```python
from build123d import *

# Parameters (mm, degrees)
SKETCH1_W           = 20
SKETCH1_H           = 20
BOSS_EXTRUDE1_DEPTH = 100
CUT_EXTRUDE1_DEPTH  = 101.995049384
CIRPATTERN1_COUNT   = 4
FILLET1_R           = 2


with BuildPart() as part:
    # Sketch1 → Boss-Extrude1 (new body)
    with BuildSketch(Plane.XY):
        Rectangle(SKETCH1_W, SKETCH1_H)
    extrude(amount=BOSS_EXTRUDE1_DEPTH)

    # Sketch2 → Cut-Extrude1 (cut, through all)
    with BuildSketch(Plane.XY):
        Polygon((6.021836642, 10), (-6.021836642, 10), (-2.5, 3.9), (2.5, 3.9), align=None)
    cut_extrude1 = extrude(amount=CUT_EXTRUDE1_DEPTH, mode=Mode.SUBTRACT)

    # CirPattern1: Cut-Extrude1 ×4 about axis
    cirpattern1_axis = Axis((0, 0, 0), (0, 0, 1))
    for i in range(1, CIRPATTERN1_COUNT):
        add(cut_extrude1.rotate(cirpattern1_axis, i * 360 / CIRPATTERN1_COUNT), mode=Mode.SUBTRACT)

    # Fillet1
    fillet1_edges = [part.edges().sort_by_distance(p)[0] for p in [
        (-10, 10, 50),
        (10, 10, 50),
        (10, -10, 50),
        (-10, -10, 50),
    ]]
    fillet(fillet1_edges, radius=FILLET1_R)


solid = part.part
```
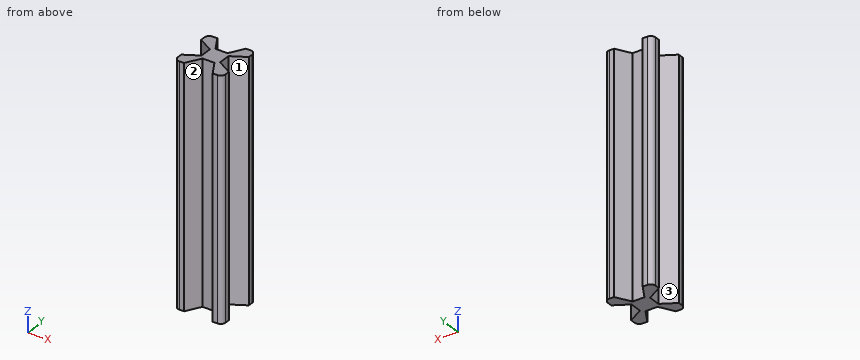
Verification items for the finished model (mm, model axes). Face numbers are marked on the shaded views. Give positions to 0.01 mm unless a question says otherwise; leave off trailing zeros. Write each loop counter-clockwise with the first axis right and the second up, starting at its lowest first coordinate (ties: lowest second). Pieces come first, ordered by that corner, then holes. Notation, with made-up numbers: M 61.25,58.25 L 95.25,58.25 A16 ccw 95.25,64.25 Z; hole C 38.25,-7 d8. An arc over 180 degrees is marked long. One line per question, with ' | ' between items.
1) Section check D-D on x = -1. Enter the section's corners in (y, z), plus the area to 3 significant figures.
Result:
outline: M -3.9,0 L 3.9,0 L 3.9,100 L -3.9,100 Z | area: 780 mm2
2) Gauge pin test, flat ends, axial feed: pin 1 Ø3 at (x, y) = (5, 7) entering from -Z; pin 2 Ø2 at (x, z) = (0, 38.5) entering from +Y; pin 3 Ø2.5 at (y, z) = (-0.5, 68.5) entering from -X; pin 4 Ø2.5 at (y, z) = (1, 48.5) entering from +X. Record the tip position at first contact, or that the pin passes through.
Result:
pin 1: stops at z = 0 | pin 2: stops at y = 3.9 | pin 3: stops at x = -3.9 | pin 4: stops at x = 3.9
3) Section check B-B on z = 17. Enter the section's corners in (x, y), plus the area to 3 significant figures.
Result:
outline: M -10,-8 A2 ccw -8,-10 L -6.02,-10 L -2.5,-3.9 L 2.5,-3.9 L 6.02,-10 L 8,-10 A2 ccw 10,-8 L 10,-6.02 L 3.9,-2.5 L 3.9,2.5 L 10,6.02 L 10,8 A2 ccw 8,10 L 6.02,10 L 2.5,3.9 L -2.5,3.9 L -6.02,10 L -8,10 A2 ccw -10,8 L -10,6.02 L -3.9,2.5 L -3.9,-2.5 L -10,-6.02 Z | area: 189 mm2
4) Section check C-C on y = 4.75. Enter the section's corners in (x, z).
Result:
outline: M -7.8,0 L -2.99,0 L -2.99,100 L -7.8,100 Z; M 2.99,0 L 7.8,0 L 7.8,100 L 2.99,100 Z
5) Mould release check, pull along X, two halves, no side actions. Record for the marked faces 1, 2 and 3: released by +X, released by -X, zero draft, split by the parting line, or undercut.
Result:
face 1: released by +X | face 2: undercut | face 3: released by -X
6) Thickness scan on line 1 along Y through (x, z) = (2.5, 54.5); line 2 along X through (y, z) = (-4, 66.5); line 3 along X through (y, z) = (-8.25, 76). Record the ranges inside material, lowest first. Write a range as [from, to].
Result:
line 1: y = [-3.9, 3.9] | line 2: x = [-6.5, -2.56], [2.56, 6.5] | line 3: x = [-9.98, -5.01], [5.01, 9.98]
7) Section check A-A on x = 5. Enter the section's corners in (y, z), plus the area to 3 significant figures.
Result:
outline: M -8.23,0 L -3.14,0 L -3.14,100 L -8.23,100 Z; M 3.14,0 L 8.23,0 L 8.23,100 L 3.14,100 Z | area: 1,020 mm2
